from build123d import *

# Parameters (mm, degrees)
F1_DEPTH = 1.5
F2_R     = 5
F3_R     = 1


with BuildPart() as f1:
    # F0 (on Front) → F1 (new body)
    with BuildSketch(Plane.XZ):
        with BuildLine():
            Line((14.275201, 0), (0, 0))
            ThreePointArc((0, 0), (-8.047761, -35.470172), (-20.547462, -69.626534))
            Line((-20.547462, -69.626534), (0, -65))
            Line((0, -65), (14.275201, -19.70393))
            Line((14.275201, -19.70393), (14.275201, 0))
        make_face()
    extrude(amount=F1_DEPTH)

    # F2
    f2_edges = [f1.edges().sort_by_distance(p)[0] for p in [
        (-20.547462, -0.75, -69.626534),
        (0, -0.75, -65),
        (14.275201, -0.75, -19.70393),
        (14.275201, -0.75, 0),
        (0, -0.75, 0),
    ]]
    fillet(f2_edges, radius=F2_R)

    # F3
    f3_edges = [f1.edges().sort_by_distance(p)[0] for p in [
        (-7.292111, 0, -32.863957),
    ]]
    fillet(f3_edges, radius=F3_R)


solid = f1.part
Part model, mm, in its own coordinate system. Coordinates: 2 decimals unless noted, no trailing zeros. Order: outer loops, then holes, each group sorted by start corner. A loop starts at its lowest first (then second) coordinate and runs counter-clockwise, first axis right, second up. Notation, with made-up numbers: M 79,58.5 L 90,58.5 A26 cw 90,90.5 Z; hole C 37,26 d10. An arc over 180 degrees is marked long. One line per question, with ' | ' between items.
Q1. Slice it at A-A (y = -0.5). Give the cut face in (x, z), and give its area (3 significant figures).
A:
outline: M -16.7,-60.81 A4.87 ccw -11.11,-67.36 L -2.84,-65.5 A4.87 ccw 0.74,-62.22 L 13.92,-20.4 A4.87 ccw 14.14,-18.93 L 14.14,-5 A4.87 ccw 9.28,-0.13 L 4.23,-0.13 A4.87 ccw -0.56,-4.16 A285.13 cw Z | area: 1,110 mm^2
Q2. Two-plate mould, pull along Y, no slides. Class faces 1 (the face through (12.772, -1.253, -1.426)), 2 (the face through (2, -1.5, -33)), 3 (the face through (-6.95, -0.29, -66.26)): +Y half, -Y half, draft (parallel to the pull), parting line (faces both ways), or undercut.
A:
face 1: draft | face 2: -Y half | face 3: +Y half
Q3. Drill centre lines: line 1 (X direction, y = -0.35, z = -60); line 2 (Y direction, x = 5.5, z = -45.5); line 3 (X direction, y = -1.4, z = -18.5). Where is each one in solid material? Low to high.
A:
line 1: x = -16.26 to 1.32 | line 2: y = -1.5 to -0.08 | line 3: x = -3.6 to 14.28
